Can you work these out from the model? Positions are in its coordinate system, mm. A direction names the side the tool comes from. Round coordinates to 2 decimals unless told otherwise and drop trailing zeros. Loops run counter-clockwise (first coordinate to the right, second up) from the corner with the lowest first, then second, coordinate; pieces in that order, holes last. Notation, with made-up numbers: (39.25, 71) -> (85.25, 71) arc R15 cw to (85.25, 83) -> close; hole circle Ø9 at (-21.5, -31). An arc over 180 degrees is marked (long way). Use a Markdown table: item, result.
from build123d import *

# Parameters (mm, degrees)
BOSS_EXTRUDE1_DEPTH = 5
BOSS_EXTRUDE2_DEPTH = 185
BOSS_EXTRUDE3_DEPTH = 5
FILLET1_R           = 10
FILLET2_R           = 2


with BuildPart() as part:
    # Sketch1 → Boss-Extrude1 (new body)
    with BuildSketch(Plane.XY):
        with BuildLine():
            Line((-71.25, 13), (-71.25, -13))
            Line((-71.25, -13), (71.25, -13))
            Line((71.25, -13), (71.25, 13))
            Line((71.25, 13), (15, 13))
            ThreePointArc((15, 13), (0, -2), (-15, 13))
            Line((-15, 13), (-71.25, 13))
        make_face()
    extrude(amount=-BOSS_EXTRUDE1_DEPTH)

    # Sketch2 → Boss-Extrude2 (add)
    with BuildSketch(Plane(origin=(0, 0, -5), x_dir=(-1, 0, 0), z_dir=(0, 0, -1))):
        Polygon((-66.25, -8), (-66.25, 8), (-66.25, 13), (-71.25, 13), (-71.25, -13), (71.25, -13), (71.25, 13), (66.25, 13), (66.25, 8), (66.25, -8), align=None)
    extrude(amount=BOSS_EXTRUDE2_DEPTH)

    # Sketch3 → Boss-Extrude3 (add)
    with BuildSketch(Plane(origin=(0, 0, -190), x_dir=(-1, 0, 0), z_dir=(0, 0, -1))):
        with BuildLine():
            Line((-66.25, 13), (-66.25, -8))
            Line((-66.25, -8), (66.25, -8))
            Line((66.25, -8), (66.25, 13))
            Line((66.25, 13), (15, 13))
            ThreePointArc((15, 13), (0, -2), (-15, 13))
            Line((-15, 13), (-66.25, 13))
        make_face()
        with BuildLine():
            Line((15, 13), (-15, 13))
            ThreePointArc((-15, 13), (0, -2), (15, 13))
        make_face()
        Polygon((71.25, 13), (66.25, 13), (66.25, -8), (-66.25, -8), (-66.25, 13), (-71.25, 13), (-71.25, -13), (71.25, -13), align=None)
    extrude(amount=BOSS_EXTRUDE3_DEPTH)

    # Fillet1
    fillet1_edges = [part.edges().sort_by_distance(p)[0] for p in [
        (71.25, -13, -97.5),
        (-71.25, -13, -97.5),
        (-15, 13, -2.5),
        (15, 13, -2.5),
        (-66.25, 2.5, -190),
        (66.25, 2.5, -190),
        (-66.25, 2.5, -5),
        (66.25, 2.5, -5),
        (71.25, 0, -195),
        (0, -13, -195),
        (-71.25, 0, -195),
        (71.25, 0, 0),
        (0, -13, 0),
        (-71.25, 0, 0),
    ]]
    fillet(fillet1_edges, radius=FILLET1_R)

    # Fillet2
    fillet2_edges = [part.edges().sort_by_distance(p)[0] for p in [
        (68.321067812, 13, -192.071067812),
        (-68.321067812, 13, -192.071067812),
        (42.081439237, 13, 0),
        (0, -2, 0),
        (-42.081439237, 13, 0),
        (-17.4356529, 11.366600265, 0),
        (17.4356529, 11.366600265, 0),
        (0, 13, -195),
        (71.25, 13, -97.5),
        (-71.25, 13, -97.5),
        (-68.321067812, 13, -2.928932188),
        (68.321067812, 13, -2.928932188),
    ]]
    fillet(fillet2_edges, radius=FILLET2_R)


solid = part.part
1. I need wall thicknesses on line 1 (X direction, y = 8, z = -108); line 2 (Z direction, x = 27, y = 4.5); line 3 (Z direction, x = -56, y = -9). Which ranges of each line are inside material? Lowest first, please.
Answer sheet:
| item | result |
|---|---|
| line 1 | x = -71.25 to -66.25, 66.25 to 71.25 |
| line 2 | z = -195 to -190, -5 to 0 |
| line 3 | z = -193 to -2 |
2. I want a section at B-B (x = 48.5). Please give me the cut outline in (y, z), plus the area to 3 significant figures.
Answer sheet:
| item | result |
|---|---|
| outline | (-13, -185) arc R10 ccw to (-3, -195) -> (11, -195) arc R2 ccw to (13, -193) -> (13, -190) -> (-8, -190) -> (-8, -5) -> (13, -5) -> (13, -2) arc R2 ccw to (11, 0) -> (-3, 0) arc R10 ccw to (-13, -10) -> close |
| area | 1,140 mm² |
3. If we mould it in two halves opening along X, with no side actions, what happens to faces 1 (the cylindrical face through (-68.4, 4.1, -191.99)), 2 (the flat face through (71.25, 4, -96)), 3 (the cylindrical face through (17.368, 11.322, -3.521)), 4 (the flat face through (-40, 4, 0))? For each: +X half, -X half, draft (parallel to the pull), parting line (faces both ways), or undercut.
Answer sheet:
| item | result |
|---|---|
| face 1 | -X half |
| face 2 | +X half |
| face 3 | undercut |
| face 4 | draft |
4. Which directions (+Z, -Z, +X, -X, +Y, -Y) give clear straight access to the entire face, cutting with the end or side of a thin tool? Please do faces 5 (the cylindrical face through (68.4, 3.9, -191.99)), 6 (the cylindrical face through (-17.368, 11.322, -3.521)), 7 (the flat face through (1, 3, -190)).
Answer sheet:
| item | result |
|---|---|
| face 5 | -Z, +X, +Y, -Y |
| face 6 | +Z, +Y |
| face 7 | +Y |
5. Will these pins go through, and if not, where does the flat tip stop? pin 1 Ø1.5 at (x, z) = (-8, -96.5) entering from +Y; pin 2 Ø3 at (y, z) = (-6.5, -26) entering from +X; pin 3 Ø6 at (x, y) = (-40, -7.5) entering from -Z; pin 4 Ø8 at (x, y) = (30.5, -2.5) entering from +Z.
Answer sheet:
| item | result |
|---|---|
| pin 1 | stops at y = -8 |
| pin 2 | stops at x = 71.05 |
| pin 3 | stops at z = -194.89 |
| pin 4 | stops at z = 0 |
6. I want a section at A-A (z = -56.5). Please give me the cut outline in (x, y).
Answer sheet:
| item | result |
|---|---|
| outline | (-71.25, -3) arc R10 ccw to (-61.25, -13) -> (61.25, -13) arc R10 ccw to (71.25, -3) -> (71.25, 11) arc R2 ccw to (69.25, 13) -> (66.25, 13) -> (66.25, -8) -> (-66.25, -8) -> (-66.25, 13) -> (-69.25, 13) arc R2 ccw to (-71.25, 11) -> close |
